The listing builds one solid part. Answer for the finished solid, in the listing's coordinates (mm). A direction names the side the tool comes from. Coordinates: 2 decimals unless noted, no trailing zeros. Order: outer loops, then holes, each group sorted by start corner. A loop starts at its lowest first (then second) coordinate and runs counter-clockwise, first axis right, second up. Notation, with made-up numbers: (43.25, 48.25) -> (78.25, 48.25) arc R35 cw to (78.25, 83.25) -> close; hole circle Ø9 at (83.5, 22). An arc over 180 degrees is marked (long way). One line per question, with ' | ' between items.
from build123d import *

# Parameters (mm, degrees)
SKETCH_1_W          = 18
SKETCH_1_H          = 34
SKETCH_1_W_2        = 14
SKETCH_1_H_2        = 24
EXTRUDE_1_DEPTH     = 10
SKETCH_2_R          = 1.1
CUT_EXTRUDE_1_DEPTH = 22.679483389
SKETCH_4_W          = 4
SKETCH_4_H          = 10
CUT_EXTRUDE_2_DEPTH = 10


with BuildPart() as part:
    # 草图1 → 凸台-拉伸1 (new body)
    with BuildSketch(Plane(origin=(0, 0, 0), x_dir=(1, 0, 0), z_dir=(0, 1, 0))):
        Rectangle(SKETCH_1_W, SKETCH_1_H)
        Rectangle(SKETCH_1_W_2, SKETCH_1_H_2, mode=Mode.SUBTRACT)
    extrude(amount=EXTRUDE_1_DEPTH)

    # 草图2 → 切除-拉伸1 (cut, through all)
    with BuildSketch(Plane.XZ):
        with Locations(Location((0, 14, 0), (0, 0, 270))):
            Circle(SKETCH_2_R)
        with Locations(Location((0, -14, 0), (0, 0, 90))):
            Circle(SKETCH_2_R)
    extrude(amount=-CUT_EXTRUDE_1_DEPTH, mode=Mode.SUBTRACT)

    # 草图4 → 切除-拉伸2 (cut)
    with BuildSketch(Plane.XY.offset(17)):
        with Locations((0, 5)):
            Rectangle(SKETCH_4_W, SKETCH_4_H)
    extrude(amount=-CUT_EXTRUDE_2_DEPTH, mode=Mode.SUBTRACT)


solid = part.part
Item 1: Section A-A, the plane x = -6 is taken. Give the vertices of the cut face in (y, z).
Computed values:
outline: (0, -17) -> (10, -17) -> (10, -12) -> (0, -12) -> close; (0, 12) -> (10, 12) -> (10, 17) -> (0, 17) -> close
Item 2: Section C-C, the plane y = 4 is taken. Give the vertices of the cut face in (x, z).
Computed values:
outline: (-9, -17) -> (9, -17) -> (9, 17) -> (2, 17) -> (2, 12) -> (7, 12) -> (7, -12) -> (-7, -12) -> (-7, 12) -> (-2, 12) -> (-2, 17) -> (-9, 17) -> close; hole circle Ø2.2 at (0, -14)
Item 3: This flat-tipped pin is pushed along its axis until it touches: pin 1 Ø3.5 at (x, z) = (0, -14) entering from -Y. Where does it stop, or does it pass through?
Computed values:
pin 1: stops at y = 0
Item 4: Section B-B, the plane z = 11.5 is taken. Give the vertices of the cut face in (x, y), plus the area to 3 significant figures.
Computed values:
outline: (-9, 0) -> (-7, 0) -> (-7, 10) -> (-9, 10) -> close; (7, 0) -> (9, 0) -> (9, 10) -> (7, 10) -> close | area: 40.0 mm^2
Item 5: For faces 1 (the face through (-7, 5, 0)), 2 (the face through (2, 5, 15)), 3 (the face through (5, 5, 17)), determine the directions among +Z, -Z, +X, -X, +Y, -Y from which every point of the face is accessible in a straight line to the end or side of a thin tool.
Computed values:
face 1: +Y, -Y | face 2: +Z, +Y, -Y | face 3: +Z, +X, -X, +Y, -Y
Item 6: Determine the mould class of faces 4 (the face through (-2, 5, 15)), 5 (the face through (-5, 5, 12)), 6 (the face through (0, 5, -17)), 7 (the face through (-6, 5, 17)) for opening direction Z: pulls with the +Z half, pulls with the -Z half, needs draft (parallel to the pull), parting line crosses it, or undercut.
Computed values:
face 4: needs draft | face 5: undercut | face 6: pulls with the -Z half | face 7: pulls with the +Z half
Item 7: Find the intervals of material crossed by L1, parallel to X at y = 8.5, z = -2; L2, parallel to X at y = 5.5, z = -14; L3, parallel to Z at x = 5.5, y = 8.5, in increasing order.
Computed values:
L1: x = -9 to -7, 7 to 9 | L2: x = -9 to -1.1, 1.1 to 9 | L3: z = -17 to -12, 12 to 17
